from build123d import *
from OCP.BRepAlgoAPI import BRepAlgoAPI_Cut
from OCP.TopTools import TopTools_ListOfShape

# Parameters (mm, degrees)
BOSS_EXTRUDE7_DEPTH     = 20.6375
SKETCH1_18_R            = 14.2875
SKETCH1_18_R_2          = 6.35
SKETCH1_18_R_3          = 34.925
SKETCH1_18_R_4          = 22.225
BOSS_EXTRUDE10_DEPTH    = 6.746875
BOSS_EXTRUDE11_START    = 6.746875
SKETCH1_20_R            = 34.925
SKETCH1_20_R_2          = 22.225
BOSS_EXTRUDE11_DEPTH    = 6.746875
BOSS_EXTRUDE12_START    = 13.692187
SKETCH1_21_R            = 14.2875
SKETCH1_21_R_2          = 6.35
SKETCH1_21_R_3          = 34.925
SKETCH1_21_R_4          = 22.225
BOSS_EXTRUDE12_DEPTH    = 6.945312
BOSS_EXTRUDE13_START    = 39.09219
SKETCH1_22_R            = 14.2875
SKETCH1_22_R_2          = 6.35
BOSS_EXTRUDE13_DEPTH    = 25.4
BOSS_EXTRUDE14_START    = 13.692187
SKETCH1_23_R            = 34.925
SKETCH1_23_R_2          = 22.225
BOSS_EXTRUDE14_DEPTH    = 19.367501
CUT_EXTRUDE3_DEPTH      = 111.865374
SKETCH5_R               = 3.175
CUT_EXTRUDE4_DEPTH      = 105.575057
CUT_EXTRUDE5_DEPTH      = 105.575057
CUT_EXTRUDE5_DEPTH_BACK = 105.575057
SKETCH6_W               = 33.02
SKETCH6_H               = 6.746875


with BuildPart() as part:
    # Sketch1 → Boss-Extrude7 (new body)
    with BuildSketch(Plane.XY):
        Polygon((38.1, 30.797578), (38.1, -30.797578), (43.65625, -30.1625), (42.588827, -25.538982), (65.327211, -6.459212), (69.85, 0), (65.327211, 6.459212), (42.588827, 25.538982), (43.65625, 30.1625), align=None)
    extrude(amount=-BOSS_EXTRUDE7_DEPTH)

    # Sketch1<18> → Boss-Extrude10 (add)
    # profile 1 of 5: a face of its own
    with BuildSketch(Plane.XY):
        with BuildLine():
            ThreePointArc((34.925, 0), (26.060233, -23.251234), (3.966094, -34.699074))
            Line((3.966094, -34.699074), (38.1, -30.797578))
            Line((38.1, -30.797578), (38.1, 30.797578))
            Line((38.1, 30.797578), (3.966094, 34.699074))
            ThreePointArc((3.966094, 34.699074), (26.060233, 23.251234), (34.925, 0))
        make_face()
    # profile 2 of 5: a face of its own
    with BuildSketch(Plane.XY):
        with BuildLine():
            Line((-55.5625, 15.014068), (-55.5625, -15.014068))
            Line((-55.5625, -15.014068), (-31.10852, -15.875))
            ThreePointArc((-31.10852, -15.875), (-34.925, 0), (-31.10852, 15.875))
            Line((-31.10852, 15.875), (-55.5625, 15.014068))
        make_face()
    # profile 3 of 5: a face of its own
    with BuildSketch(Plane.XY):
        with BuildLine():
            ThreePointArc((-61.9125, 0), (-66.097212, -10.102788), (-76.2, -14.2875))
            Line((-76.2, -14.2875), (-55.5625, -15.014068))
            Line((-55.5625, -15.014068), (-55.5625, 15.014068))
            Line((-55.5625, 15.014068), (-76.2, 14.2875))
            ThreePointArc((-76.2, 14.2875), (-66.097212, 10.102788), (-61.9125, 0))
        make_face()
    # profile 4 of 5: a face of its own
    with BuildSketch(Plane.XY):
        with Locations((-76.2, 0)):
            Circle(SKETCH1_18_R)
        with Locations((-76.2, 0)):
            Circle(SKETCH1_18_R_2, mode=Mode.SUBTRACT)
    # profile 5 of 5: a face of its own
    with BuildSketch(Plane.XY):
        Circle(SKETCH1_18_R_3)
        Circle(SKETCH1_18_R_4, mode=Mode.SUBTRACT)
    extrude(amount=-BOSS_EXTRUDE10_DEPTH)

    # Sketch1<20> → Boss-Extrude11 (add)
    # profile 1 of 5: a face of its own
    with BuildSketch(Plane.XY.offset(BOSS_EXTRUDE11_START)):
        Circle(SKETCH1_20_R)
        Circle(SKETCH1_20_R_2, mode=Mode.SUBTRACT)
    # profile 2 of 5: a face of its own
    with BuildSketch(Plane.XY.offset(BOSS_EXTRUDE11_START)):
        with BuildLine():
            ThreePointArc((34.925, 0), (26.060233, -23.251234), (3.966094, -34.699074))
            Line((3.966094, -34.699074), (38.1, -30.797578))
            Line((38.1, -30.797578), (38.1, 30.797578))
            Line((38.1, 30.797578), (3.966094, 34.699074))
            ThreePointArc((3.966094, 34.699074), (26.060233, 23.251234), (34.925, 0))
        make_face()
    # profile 3 of 5: a face of its own
    with BuildSketch(Plane.XY.offset(BOSS_EXTRUDE11_START)):
        Polygon((38.1, 30.797578), (38.1, -30.797578), (43.65625, -30.1625), (42.588827, -25.538982), (47.625, -21.313131), (47.625, 21.313131), (42.588827, 25.538982), (43.65625, 30.1625), align=None)
    # profile 4 of 5: a face of its own
    with BuildSketch(Plane.XY.offset(BOSS_EXTRUDE11_START)):
        with BuildLine():
            Line((-55.5625, 15.014068), (-55.5625, -15.014068))
            Line((-55.5625, -15.014068), (-31.10852, -15.875))
            ThreePointArc((-31.10852, -15.875), (-34.925, 0), (-31.10852, 15.875))
            Line((-31.10852, 15.875), (-55.5625, 15.014068))
        make_face()
    # profile 5 of 5: a face of its own
    with BuildSketch(Plane.XY.offset(BOSS_EXTRUDE11_START)):
        with BuildLine():
            ThreePointArc((-61.9125, 0), (-66.097212, -10.102788), (-76.2, -14.2875))
            Line((-76.2, -14.2875), (-55.5625, -15.014068))
            Line((-55.5625, -15.014068), (-55.5625, 15.014068))
            Line((-55.5625, 15.014068), (-76.2, 14.2875))
            ThreePointArc((-76.2, 14.2875), (-66.097212, 10.102788), (-61.9125, 0))
        make_face()
    extrude(amount=-BOSS_EXTRUDE11_DEPTH)

    # Sketch1<21> → Boss-Extrude12 (add)
    # profile 1 of 6: a face of its own
    with BuildSketch(Plane.XY.offset(BOSS_EXTRUDE12_START)):
        with Locations((-76.2, 0)):
            Circle(SKETCH1_21_R)
        with Locations((-76.2, 0)):
            Circle(SKETCH1_21_R_2, mode=Mode.SUBTRACT)
    # profile 2 of 6: a face of its own
    with BuildSketch(Plane.XY.offset(BOSS_EXTRUDE12_START)):
        with BuildLine():
            ThreePointArc((-61.9125, 0), (-66.097212, -10.102788), (-76.2, -14.2875))
            Line((-76.2, -14.2875), (-55.5625, -15.014068))
            Line((-55.5625, -15.014068), (-55.5625, 15.014068))
            Line((-55.5625, 15.014068), (-76.2, 14.2875))
            ThreePointArc((-76.2, 14.2875), (-66.097212, 10.102788), (-61.9125, 0))
        make_face()
    # profile 3 of 6: a face of its own
    with BuildSketch(Plane.XY.offset(BOSS_EXTRUDE12_START)):
        with BuildLine():
            Line((-55.5625, 15.014068), (-55.5625, -15.014068))
            Line((-55.5625, -15.014068), (-31.10852, -15.875))
            ThreePointArc((-31.10852, -15.875), (-34.925, 0), (-31.10852, 15.875))
            Line((-31.10852, 15.875), (-55.5625, 15.014068))
        make_face()
    # profile 4 of 6: a face of its own
    with BuildSketch(Plane.XY.offset(BOSS_EXTRUDE12_START)):
        Circle(SKETCH1_21_R_3)
        Circle(SKETCH1_21_R_4, mode=Mode.SUBTRACT)
    # profile 5 of 6: a face of its own
    with BuildSketch(Plane.XY.offset(BOSS_EXTRUDE12_START)):
        with BuildLine():
            ThreePointArc((34.925, 0), (26.060233, -23.251234), (3.966094, -34.699074))
            Line((3.966094, -34.699074), (38.1, -30.797578))
            Line((38.1, -30.797578), (38.1, 30.797578))
            Line((38.1, 30.797578), (3.966094, 34.699074))
            ThreePointArc((3.966094, 34.699074), (26.060233, 23.251234), (34.925, 0))
        make_face()
    # profile 6 of 6: a face of its own
    with BuildSketch(Plane.XY.offset(BOSS_EXTRUDE12_START)):
        Polygon((38.1, 30.797578), (38.1, -30.797578), (43.65625, -30.1625), (42.588827, -25.538982), (47.625, -21.313131), (47.625, 21.313131), (42.588827, 25.538982), (43.65625, 30.1625), align=None)
    extrude(amount=-BOSS_EXTRUDE12_DEPTH)


with BuildPart() as boss_extrude13_tool:
    # Sketch1<22> → Boss-Extrude13 (new body)
    with BuildSketch(Plane.XY.offset(BOSS_EXTRUDE13_START)):
        with Locations(Location((-76.2, 0, 0), (0, 0, 270))):
            Circle(SKETCH1_22_R)
        with Locations((-76.2, 0)):
            Circle(SKETCH1_22_R_2, mode=Mode.SUBTRACT)
    extrude(amount=-BOSS_EXTRUDE13_DEPTH)


with BuildPart() as part_1:
    add(part.part)


with BuildPart() as part_2:
    # Boss-Extrude13: joined with boss_extrude13_tool
    add(part_1.part.fuse(boss_extrude13_tool.part, tol=0.00001))

    # Sketch1<23> → Boss-Extrude14 (add)
    with BuildSketch(Plane.XY.offset(BOSS_EXTRUDE14_START)):
        Circle(SKETCH1_23_R)
        Circle(SKETCH1_23_R_2, mode=Mode.SUBTRACT)
    extrude(amount=BOSS_EXTRUDE14_DEPTH)


with BuildPart() as cut_extrude3_tool:
    # Sketch4 → Cut-Extrude3 (new, through all)
    with BuildSketch(Plane.XY.offset(33.059687)):
        with BuildLine():
            Line((0, -23.38371), (0, -22.225))
            ThreePointArc((0, -22.225), (-0.595526, -22.21702), (-1.190625, -22.193085))
            Line((-1.190625, -22.193085), (-1.190625, -23.38371))
            Line((-1.190625, -23.38371), (0, -23.38371))
        make_face()
        with BuildLine():
            ThreePointArc((1.190625, -22.193085), (0.595526, -22.21702), (0, -22.225))
            Line((0, -22.225), (0, -23.38371))
            Line((0, -23.38371), (1.190625, -23.38371))
            Line((1.190625, -23.38371), (1.190625, -22.193085))
        make_face()
    extrude(amount=-CUT_EXTRUDE3_DEPTH)


with BuildPart() as part_3:
    add(part_2.part)

    # Cut-Extrude3: cut by cut_extrude3_tool, with a tolerance
    cut_extrude3_stock = TopTools_ListOfShape()
    cut_extrude3_stock.Append(part_3.part.wrapped)
    cut_extrude3_tools = TopTools_ListOfShape()
    cut_extrude3_tools.Append(cut_extrude3_tool.part.wrapped)
    cut_extrude3_cut = BRepAlgoAPI_Cut()
    cut_extrude3_cut.SetArguments(cut_extrude3_stock)
    cut_extrude3_cut.SetTools(cut_extrude3_tools)
    cut_extrude3_cut.SetFuzzyValue(0.00001)
    cut_extrude3_cut.Build()
    add(Compound.cast(cut_extrude3_cut.Shape()).solids(), mode=Mode.REPLACE)

    # Sketch5 → Cut-Extrude4 (cut, through all)
    with BuildSketch(Plane(origin=(0, 0, 0), x_dir=(1, 0, 0), z_dir=(0, 1, 0))):
        with Locations(Location((0, -13.156406, 0), (0, 0, 270))):
            Circle(SKETCH5_R)
    extrude(amount=-CUT_EXTRUDE4_DEPTH, mode=Mode.SUBTRACT)

    # Sketch6 → Cut-Extrude5 (cut, two sides: drawn at the far end of the back side and taken through both)
    with BuildSketch(Plane(origin=(0, 0, 0), x_dir=(1, 0, 0), z_dir=(0, 1, 0)).offset(-CUT_EXTRUDE5_DEPTH_BACK)):
        with Locations((-73.9775, -3.373437)):
            Rectangle(SKETCH6_W, SKETCH6_H)
    extrude(amount=CUT_EXTRUDE5_DEPTH + CUT_EXTRUDE5_DEPTH_BACK, mode=Mode.SUBTRACT)


solid = part_3.part
The model under review builds one solid part; all positions refer to its coordinate system, in mm. A direction names the side the tool comes from. Round coordinates to 2 decimals unless told otherwise and drop trailing zeros. Loops run counter-clockwise (first coordinate to the right, second up) from the corner with the lowest first, then second, coordinate; pieces in that order, holes last. Notation, with made-up numbers: (23.25, 6.5) -> (52.25, 6.5) arc R29 ccw to (52.25, 34.5) -> close; hole circle Ø2 at (-27, 66.5). An arc over 180 degrees is marked (long way). Write item = value, one per line. Start each with the question number.
Item 1: Take a section at A-A on z = 26. Count the separate pieces of the cut face and the enclosed holes in it, plus the area to 3 significant figures.
Item 2: Take a section at D-D on x = -6. Give the boundary of the cut face in (y, z), plus the area to 3 significant figures.
Item 3: For faces 1 (the cylindrical face through (-90.148, 3.097, 23.146)), 2 (the cylindrical face through (-2.817, -28.372, 14.621)), 3 (the flat face through (-27, 0, -6.747)), 4 (the flat face through (-57.468, 0, 3)), 5 (the flat face through (47.625, 0, 7)), list the 3-axis set-ups (+Z, -Z, +X, -X, +Y, -Y) from which the entire face can be reached by the end or side of a thin tool; tool diameter is ignored.
Item 4: To check wall thickness, follow L1, parallel to Z at x = 0, y = -26.25; L2, parallel to Y at x = -76, z = -3; L3, parallel to Y at x = 0, z = 22 (3 decimals). State the ranges of each line that lie inside material, in increasing order.
Item 5: Insertion check: pin 1 (6 mm diameter, centred on y = -20, z = -8.5, fed in from -X); pin 2 (4 mm diameter, centred on x = 34.5, y = -2.5, fed in from -Z); pin 3 (3.5 mm diameter, centred on y = 0, z = 3, fed in from -X). Each pin has a flat end and moves straight along its axis. Give the tip position at first contact, or say it passes through.
Item 6: Mouldability with a two-part tool opening along X and no side actions: class faces 6 (the flat face through (43.13, -27.88, -3.23)), 7 (the flat face through (-79, -6, 39.092)), 8 (the cylindrical face through (-82.544, 0.279, -3.326)) as released by +X, released by -X, zero draft, split by the parting line, or undercut.
Item 7: Take a section at C-C on z = -8.5. Give the boundary of the cut face in (x, y), plus the area to 3 significant figures.
Result:
q1.separate_pieces = 2
q1.enclosed_holes = 2
q1.area = 2,790 mm²
q2.outline = (-34.41, -6.75) -> (-21.4, -6.75) -> (-21.4, 33.06) -> (-34.41, 33.06) -> close; (21.4, -6.75) -> (34.41, -6.75) -> (34.41, 33.06) -> (21.4, 33.06) -> close
q2.area = 1,040 mm²
q3.face_1 = +Z
q3.face_2 = -Y
q3.face_3 = -Z, -X, +Y, -Y
q3.face_4 = -X, +Y, -Y
q3.face_5 = +Z, +X, +Y, -Y
q4.L1 = -6.75 to 9.98, 16.33 to 33.06
q4.L2 = -14.29 to -6.35, 6.35 to 14.29
q4.L3 = -34.925 to -23.384, 22.225 to 34.925
q5.pin_1 = -30.19
q5.pin_2 = -6.75
q5.pin_3 = -57.47
q6.face_6 = released by +X
q6.face_7 = zero draft
q6.face_8 = undercut
q7.outline = (38.1, -30.8) -> (43.66, -30.16) -> (42.59, -25.54) -> (65.33, -6.46) -> (69.85, 0) -> (65.33, 6.46) -> (42.59, 25.54) -> (43.66, 30.16) -> (38.1, 30.8) -> close
q7.area = 1,040 mm²
